Part model, mm, in its own coordinate system. Coordinates: 2 decimals unless noted, no trailing zeros. Loops run counter-clockwise (first coordinate to the right, second up) from the corner with the lowest first, then second, coordinate; pieces in that order, holes last. Notation, with made-up numbers: M 87,-21.75 L 127,-21.75 A12 ccw 127,-0.75 Z; hole C 54.25,65.5 d3. An arc over 180 degrees is marked long. Use a Markdown table: item, result. Add a question column.
1) Band-saw the part on D-D (y = -8). List the corners of the cut face in (x, z).
2) Band-saw the part on B-B (z = 2.5). List the corners of the cut face in (x, y), plus the area to 3 significant figures.
3) Pin check, flat tips, straight feed: pin 1 Ø4 at (y, z) = (-5, 1) entering from +X; pin 2 Ø2 at (y, z) = (-9.5, 2.5) entering from +X; pin 3 Ø2 at (y, z) = (-6, 3) entering from -X. Stop position of each tip, or through.
4) Wall check: probe 1 along Y at (x, z) = (10.5, 1); probe 2 along X at (y, z) = (-19.5, 3.5); probe 3 along X at (y, z) = (22, 3.5). Give the ranges that are in metal, low to high. Write a range as from..to.
5) Pull direction Y, two halves, no side cores. Call faces 1 (the cylindrical face through (8.136, 10.145, 3.993)), 2 (the flat face through (-27.627, 21.901, 3.993)), 3 (the flat face through (6, 9, 0)), 4 (the cylindrical face through (-21.546, 21.418, 3.993)): released by +Y, released by -Y, zero draft, split by the parting line, or undercut.
6) Band-saw the part on C-C (x = -19). List the corners of the cut face in (y, z).
7) Band-saw the part on A-A (y = 9). List the corners of the cut face in (x, z).
from build123d import *

# Parameters (mm, degrees)
SKETCH_1_R      = 1.8
EXTRUDE_1_DEPTH = 8.1


with BuildPart() as part:
    # 草图1 → 凸台-拉伸1 (new body)
    with BuildSketch(Plane.XY):
        with BuildLine():
            Line((-28.085321485, 24.455311821), (-27.156538847, 19.274809777))
            ThreePointArc((-27.156538847, 19.274809777), (-26.008495854, 17.407885349), (-23.897169242, 16.819914712))
            ThreePointArc((-23.897169242, 16.819914712), (6.047612353, 6.174156813), (16.688201762, -23.772461744))
            ThreePointArc((16.688201762, -23.772461744), (17.279148071, -25.888317514), (19.153455893, -27.034194196))
            Line((19.153455893, -27.034194196), (24.335957665, -27.944492213))
            ThreePointArc((24.335957665, -27.944492213), (26.653907402, -27.390513858), (27.836563196, -25.321429936))
            ThreePointArc((27.836563196, -25.321429936), (13.995899045, 14.135772324), (-25.464877169, 27.96624357))
            ThreePointArc((-25.464877169, 27.96624357), (-27.536589514, 26.779128998), (-28.085321485, 24.455311821))
        make_face()
        with Locations((22.382403744, -19.986536191)):
            Circle(SKETCH_1_R, mode=Mode.SUBTRACT)
        with Locations((9.934441945, 10.06550201)):
            Circle(SKETCH_1_R, mode=Mode.SUBTRACT)
        with Locations((-20.117596256, 22.513463809)):
            Circle(SKETCH_1_R, mode=Mode.SUBTRACT)
    extrude(amount=EXTRUDE_1_DEPTH)


solid = part.part
Entries:
| question | item | result |
|---|---|---|
| 1 | outline | M 14.89,0 L 26.62,0 L 26.62,8.1 L 14.89,8.1 Z |
| 2 | outline | M -28.09,24.46 L -27.16,19.27 A3 ccw -23.9,16.82 A37 cw 16.69,-23.77 A3 ccw 19.15,-27.03 L 24.34,-27.94 A3 ccw 27.84,-25.32 A48.25 ccw -25.46,27.97 A3 ccw Z; hole C -20.12,22.51 d3.6; hole C 9.93,10.07 d3.6; hole C 22.38,-19.99 d3.6 |
| 2 | area | 885 mm2 |
| 3 | pin 1 | x = 26.35 |
| 3 | pin 2 | x = 27.19 |
| 3 | pin 3 | x = 13.71 |
| 4 | probe 1 | 0.79..8.36, 11.77..17.3 |
| 4 | probe 2 | 16.88..20.65, 24.12..28.13 |
| 4 | probe 3 | -27.65..-21.84, -18.39..3.66 |
| 5 | face 1 | undercut |
| 5 | face 2 | released by -Y |
| 5 | face 3 | zero draft |
| 5 | face 4 | undercut |
| 6 | outline | M 17,0 L 21.1,0 L 21.1,8.1 L 17,8.1 Z; M 23.92,0 L 28.25,0 L 28.25,8.1 L 23.92,8.1 Z |
| 7 | outline | M 2.88,0 L 8.48,0 L 8.48,8.1 L 2.88,8.1 Z; M 11.39,0 L 18.45,0 L 18.45,8.1 L 11.39,8.1 Z |
